Work out the finished part from the listing and answer in its coordinate system (mm). A direction names the side the tool comes from. Round coordinates to 2 decimals unless told otherwise and drop trailing zeros. Loops run counter-clockwise (first coordinate to the right, second up) from the corner with the lowest first, then second, coordinate; pieces in that order, holes last. Notation, with made-up numbers: (-14, 66.25) - (26, 66.25) arc R21 ccw to (26, 93.25) - close; hole circle Ø9 at (38, -25). An arc over 180 degrees is marked (long way). Use CSV: the item, a comma, the result in double quotes. Start each with the question number.
from build123d import *

# Parameters (mm, degrees)
SKETCH1_W                  = 17.2
SKETCH1_H                  = 14.4
BOSS_EXTRUDE1_DEPTH        = 18
SKETCH2_R                  = 5.875
BOSS_EXTRUDE2_DEPTH        = 13
SKETCH3_R                  = 4
BOSS_EXTRUDE3_DEPTH        = 5
SKETCH4_R                  = 5
BOSS_EXTRUDE4_DEPTH        = 5
SKETCH5_W                  = 10
SKETCH5_H                  = 7.5
BOSS_EXTRUDE5_DEPTH        = 1.2
SKETCH6_W                  = 0.8
SKETCH6_H                  = 0.8
BOSS_EXTRUDE6_DEPTH        = 7.3
CHAMFER1_SIZE              = 0.4
FILLET1_R                  = 1
FILLET2_R                  = 0.5
SKETCH7_R                  = 5.875
BOSS_EXTRUDE7_DEPTH        = 2.2
CHAMFER2_SIZE              = 0.6
LPATTERN1_COUNT            = 3
LPATTERN1_PITCH            = 7
LPATTERN1_COUNT_DIR2       = 2
LPATTERN1_PITCH_DIR2       = 9
CHAMFER1_OF_LPATTERN1_SIZE = 0.4


with BuildPart() as part:
    # Sketch1 → Boss-Extrude1 (new body)
    with BuildSketch(Plane.XY):
        with Locations((8.6, 7.2)):
            Rectangle(SKETCH1_W, SKETCH1_H)
    extrude(amount=BOSS_EXTRUDE1_DEPTH)

    # Sketch2 → Boss-Extrude2 (add)
    with BuildSketch(Plane.XY.offset(18)):
        with Locations(Location((8.6, 7.2, 0), (0, 0, 180))):
            Circle(SKETCH2_R)
    extrude(amount=BOSS_EXTRUDE2_DEPTH)

    # Sketch3 → Boss-Extrude3 (add)
    with BuildSketch(Plane.XY.offset(31)):
        with Locations((8.6, 7.2)):
            Circle(SKETCH3_R)
    extrude(amount=BOSS_EXTRUDE3_DEPTH)

    # Sketch4 → Boss-Extrude4 (add)
    with BuildSketch(Plane.XY.offset(36)):
        with Locations((8.6, 7.2)):
            Circle(SKETCH4_R)
    extrude(amount=BOSS_EXTRUDE4_DEPTH)

    # Sketch5 → Boss-Extrude5 (add)
    with BuildSketch(Plane(origin=(0, 0, 0), x_dir=(-1, 0, 0), z_dir=(0, 0, -1))):
        with Locations((-8.6, 7.2)):
            Rectangle(SKETCH5_W, SKETCH5_H)
    extrude(amount=BOSS_EXTRUDE5_DEPTH)

    # Sketch6 → Boss-Extrude6 (add)
    with BuildSketch(Plane(origin=(0, 0, 0), x_dir=(-1, 0, 0), z_dir=(0, 0, -1))):
        with Locations((-15.6, 11.7)):
            Rectangle(SKETCH6_W, SKETCH6_H)
    boss_extrude6 = extrude(amount=BOSS_EXTRUDE6_DEPTH)

    # Chamfer1
    chamfer1_edges = [part.edges().sort_by_distance(p)[0] for p in [
        (15.2, 11.7, -7.3),
        (15.6, 12.1, -7.3),
        (16, 11.7, -7.3),
        (15.6, 11.3, -7.3),
    ]]
    chamfer(chamfer1_edges, length=CHAMFER1_SIZE - 0.0001)  # a hair under: the kernel refuses the full size

    # Fillet1
    fillet1_edges = [part.edges().sort_by_distance(p)[0] for p in [
        (14.475, 7.2, 18),
    ]]
    fillet(fillet1_edges, radius=FILLET1_R)

    # Fillet2
    fillet2_edges = [part.edges().sort_by_distance(p)[0] for p in [
        (3.6, 7.2, 41),
    ]]
    fillet(fillet2_edges, radius=FILLET2_R)

    # Sketch7 → Boss-Extrude7 (add)
    with BuildSketch(Plane.XY.offset(19)):
        Polygon((16.682903769, 7.2), (12.641451884, 14.2), (4.558548116, 14.2), (0.517096231, 7.2), (4.558548116, 0.2), (12.641451884, 0.2), align=None)
        with Locations(Location((8.6, 7.2, 0), (0, 0, 180))):
            Circle(SKETCH7_R, mode=Mode.SUBTRACT)
    extrude(amount=BOSS_EXTRUDE7_DEPTH)

    # Chamfer2
    chamfer2_edges = [part.edges().sort_by_distance(p)[0] for p in [
        (14.662177826, 3.7, 21.2),
        (14.662177826, 10.7, 21.2),
        (8.6, 14.2, 21.2),
        (2.537822174, 10.7, 21.2),
        (2.537822174, 3.7, 21.2),
        (8.6, 0.2, 21.2),
        (14.662177826, 3.7, 19),
        (14.662177826, 10.7, 19),
        (8.6, 14.2, 19),
        (2.537822174, 10.7, 19),
        (2.537822174, 3.7, 19),
        (8.6, 0.2, 19),
    ]]
    chamfer(chamfer2_edges, length=CHAMFER2_SIZE)

    # LPattern1: Boss-Extrude6 3 × 2
    with Locations(*[(-i * LPATTERN1_PITCH, -j * LPATTERN1_PITCH_DIR2, 0) for i in range(LPATTERN1_COUNT) for j in range(LPATTERN1_COUNT_DIR2) if (i, j) != (0, 0)]):
        add(boss_extrude6)

    # Chamfer1 of LPattern1
    chamfer1_of_lpattern1_edges = [part.edges().sort_by_distance(p)[0] for p in [
        (15.2, 2.7, -7.3),
        (15.6, 3.1, -7.3),
        (16, 2.7, -7.3),
        (15.6, 2.3, -7.3),
        (8.2, 11.7, -7.3),
        (8.6, 12.1, -7.3),
        (9, 11.7, -7.3),
        (8.6, 11.3, -7.3),
        (8.2, 2.7, -7.3),
        (8.6, 3.1, -7.3),
        (9, 2.7, -7.3),
        (8.6, 2.3, -7.3),
        (1.2, 11.7, -7.3),
        (1.6, 12.1, -7.3),
        (2, 11.7, -7.3),
        (1.6, 11.3, -7.3),
        (1.2, 2.7, -7.3),
        (1.6, 3.1, -7.3),
        (2, 2.7, -7.3),
        (1.6, 2.3, -7.3),
    ]]
    chamfer(chamfer1_of_lpattern1_edges, length=CHAMFER1_OF_LPATTERN1_SIZE - 0.0001)  # a hair under: the kernel refuses the full size


solid = part.part
Item 1: Each of these flat-tipped pins is pushed along its axis until it touches: pin 1 Ø5 at (x, y) = (8, 2) entering from +Z; pin 2 Ø6.5 at (x, y) = (12, 5.5) entering from -Z; pin 3 Ø0.6 at (x, z) = (15.5, -2.5) entering from -Y; pin 4 Ø2 at (x, z) = (3.5, 20.5) entering from +Y. Where does it stop, or does it pass through?
Item 2: Which of the six approach directions +Z, -Z, +X, -X, +Y, -Y give full straight-line access (tool end or side, diameter ignored) to faces 4 (the flat face through (6, 11, 36)), 5 (the flat face through (15.2, 11.7, -3.4)), 6 (the flat face through (13.6, 7, -1))?
Item 3: A cutting plane is placed at B-B (z = 27). Determine the outline of the cut face in (x, y) (3 decimals), plus the area to 3 significant figures.
Item 4: The mould has two halves that part along Z. Classify faces 1 (the flat face through (2.822, 10.601, 19.304)), 2 (the flat face through (15.6, 3.1, -3.4)), 3 (the flat face through (9, 7, -1.2)): pulls with the +Z half, pulls with the -Z half, needs draft (parallel to the pull), parting line crosses it, or undercut.
Item 5: Find the intervals of material crossed by probe 1 along Z at (x, y) = (11.5, 13.5); probe 2 along Z at (x, y) = (4.5, 8.25); probe 3 along Y at (x, z) = (8.5, 35), in increasing order. Write a range as [from, to].
Item 6: A cutting plane is placed at A-A (z = 32). Determine the outline of the cut face in (x, y).
Result sheet:
1,pin 1,"z = 41"
1,pin 2,"z = -1.2"
1,pin 3,"y = 2.3"
1,pin 4,"y = 14.1"
2,face 4,"none"
2,face 5,"-Z, +Y, -Y"
2,face 6,"-Z, +X, +Y, -Y"
3,outline,"circle Ø11.75 at (8.6, 7.2)"
3,area,"108 mm^2"
4,face 1,"undercut"
4,face 2,"needs draft"
4,face 3,"pulls with the -Z half"
5,probe 1,"[0, 18], [19, 21.2]"
5,probe 2,"[-1.2, 31], [36, 41]"
5,probe 3,"[3.2, 11.2]"
6,outline,"circle Ø8 at (8.6, 7.2)"
